Could you check a few things on this model? Use its own coordinates, in mm. A direction names the side the tool comes from. Give positions to 0.01 mm unless a question says otherwise; leave off trailing zeros. Write each loop counter-clockwise with the first axis right and the second up, starting at its lowest first coordinate (ties: lowest second). Pieces come first, ordered by that corner, then holes. Notation, with made-up numbers: M 14,4 L 52,4 A3 cw 52,8 Z; hole C -30,48.25 d8. An arc over 180 degrees is marked long. One line per item, written item: value.
```python
from build123d import *

# Parameters (mm, degrees)
SKETCH1_W                   = 254
SKETCH1_H                   = 114.3
BOSS_EXTRUDE1_DEPTH         = 9.525
SKETCH2_R                   = 10
CUT_EXTRUDE1_DEPTH          = 140.5917194
F_3_8_CLEARANCE_HOLE1_D     = 9.8044
F_3_8_CLEARANCE_HOLE1_DEPTH = 10
F_3_8_CLEARANCE_HOLE1_TIP   = 2.945538927
FILLET1_R                   = 2
M3_CLEARANCE_HOLE1_D        = 3.6
M3_CLEARANCE_HOLE1_DEPTH    = 10
M3_CLEARANCE_HOLE1_TIP      = 1.081549114
CUT_EXTRUDE2_START          = -7.525
SKETCH11_R                  = 12.5
SKETCH11_R_2                = 10
CUT_EXTRUDE2_DEPTH          = 7.525


with BuildPart() as part:
    # Sketch1 → Boss-Extrude1 (new body)
    with BuildSketch(Plane(origin=(0, 0, 0), x_dir=(1, 0, 0), z_dir=(0, 1, 0))):
        Rectangle(SKETCH1_W, SKETCH1_H)
    extrude(amount=BOSS_EXTRUDE1_DEPTH)

    # Sketch2 → Cut-Extrude1 (cut, through all)
    with BuildSketch(Plane(origin=(0, 9.525, 0), x_dir=(1, 0, 0), z_dir=(0, 1, 0))):
        with Locations(Location((107.475, 0, 0), (0, 0, 270))):
            Circle(SKETCH2_R)
    extrude(amount=-CUT_EXTRUDE1_DEPTH, mode=Mode.SUBTRACT)

    # 3/8 Clearance Hole1
    with Locations(Plane(origin=(0, 9.525, 0), x_dir=(1, 0, 0), z_dir=(0, 1, 0))):
        with Locations((112.7125, 42.8625), (112.7125, -42.8675), (-112.7175, -42.8675), (-112.7175, 42.8625)):
            Hole(F_3_8_CLEARANCE_HOLE1_D / 2, depth=F_3_8_CLEARANCE_HOLE1_DEPTH)
            with Locations((0, 0, -(F_3_8_CLEARANCE_HOLE1_DEPTH + F_3_8_CLEARANCE_HOLE1_TIP / 2))):  # 118° drill point
                Cone(0, F_3_8_CLEARANCE_HOLE1_D / 2, F_3_8_CLEARANCE_HOLE1_TIP, mode=Mode.SUBTRACT)

    # Fillet1
    fillet1_edges = [part.edges().sort_by_distance(p)[0] for p in [
        (127, 4.7625, 57.15),
        (-127, 4.7625, 57.15),
        (-127, 4.7625, -57.15),
        (127, 4.7625, -57.15),
    ]]
    fillet(fillet1_edges, radius=FILLET1_R)

    # M3 Clearance Hole1
    with Locations(Plane.XZ):
        with Locations((77.95, 22.1), (77.95, -22.1)):
            Hole(M3_CLEARANCE_HOLE1_D / 2, depth=M3_CLEARANCE_HOLE1_DEPTH)
            with Locations((0, 0, -(M3_CLEARANCE_HOLE1_DEPTH + M3_CLEARANCE_HOLE1_TIP / 2))):  # 118° drill point
                Cone(0, M3_CLEARANCE_HOLE1_D / 2, M3_CLEARANCE_HOLE1_TIP, mode=Mode.SUBTRACT)

    # Sketch11 → Cut-Extrude2 (cut)
    with BuildSketch(Plane.XZ.offset(CUT_EXTRUDE2_START)):
        with Locations(Location((107.475, 0, 0), (0, 0, 270))):
            Circle(SKETCH11_R)
        with Locations(Location((107.475, 0, 0), (0, 0, 90))):
            Circle(SKETCH11_R_2, mode=Mode.SUBTRACT)
    extrude(amount=CUT_EXTRUDE2_DEPTH, mode=Mode.SUBTRACT)


solid = part.part
```
1) Please list where these lines run through material, in increasing order: L1, parallel to Z at x = 77.95, y = 6; L2, parallel to X at y = 8.5, z = -40.5; L3, parallel to Z at x = 110, y = 9. Write a range as from..to.
Outcome:
L1: z = -57.15..-23.9, -20.3..20.3, 23.9..57.15
L2: x = -127..-117.01, -108.42..108.42, 117.01..127
L3: z = -57.15..-46.95, -38.78..-9.68, 9.68..38.78, 46.95..57.15
2) If we section it at B-B, the plane y = 3.25: Give the number of separate pieces and of enclosed holes in the cut face, then the cut area to 3 significant figures.
Outcome:
separate pieces: 1
enclosed holes: 7
area: 28,200 mm^2
3) On a 3-axis mill with a long thin cutter (end or side, diameter ignored), from which of +Z, -Z, +X, -X, +Y, -Y can I reach the whole of each face in a straight line? I mean faces 5 (the face through (-117.393, 4.696, 41.395)), 6 (the face through (116, 7.525, 6)). Say none if no direction works.
Outcome:
face 5: +Y, -Y
face 6: -Y
4) I'm going to push a flat-ended pin straight in: pin 1 (6 mm diameter, centred on x = 112.71, z = -42.86, fed in from +Y). Where does the tip first touch, or does it pass through?
Outcome:
pin 1: passes through
5) We'd pull the mould along X, two halves only. Please class faces 1 (the face through (117.39, 8.54, -1.3)), 2 (the face through (127, 5, 1)), 3 (the face through (-2, 5, 57.15)), 4 (the face through (-127, 5, 1)): pulls with the +X half, pulls with the -X half, needs draft (parallel to the pull), parting line crosses it, or undercut.
Outcome:
face 1: undercut
face 2: pulls with the +X half
face 3: needs draft
face 4: pulls with the -X half
6) If we section it at A-A, the plane z = 0: Write out the boundary of the cut face in (x, y) (3 decimals).
Outcome:
outline: M -127,0 L 94.975,0 L 94.975,7.525 L 97.475,7.525 L 97.475,9.525 L -127,9.525 Z; M 117.475,7.525 L 119.975,7.525 L 119.975,0 L 127,0 L 127,9.525 L 117.475,9.525 Z
